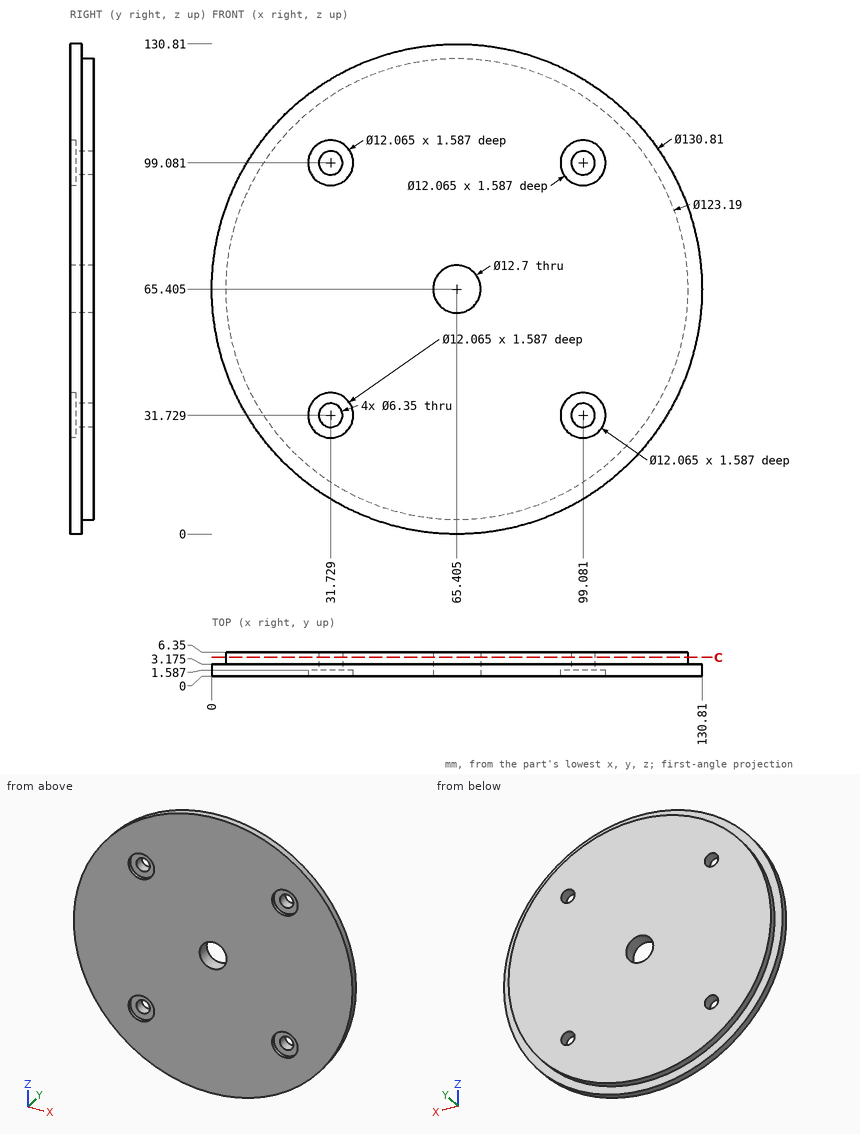
Verification items for this drawing (mm, ordinates from the low corner). Give positions to 0.01 mm unless a question says otherwise; leave off trailing zeros. Use a Markdown table: item, result.
Item 1: Section check C-C (y = 5). State how many separate pieces and enclosed holes the cut face has, and give its area (3 significant figures).
Answers follow:
| item | result |
|---|---|
| separate pieces | 1 |
| enclosed holes | 5 |
| area | 11,700 mm2 |
Item 2: Depth check by flat-ended pin: P1, Ø1.5, axis at x = 70.5, y = 4, coming from the -Z side; P2, Ø6, axis at x = 32, z = 99, coming from the -Y side. Enter the tip coordinate at first touch or a pass-through.
Answers follow:
| item | result |
|---|---|
| P1 | stops at z = 3.96 |
| P2 | stops at y = 1.59 |
Item 3: Material ranges on line 1 along Z through (x, y) = (32, 3.5) (1 decimal); line 2 along X through (y, z) = (3, 98.5); line 3 along X through (y, z) = (1.5, 64) (1 decimal), recorded low to high.
Answers follow:
| item | result |
|---|---|
| line 1 | z = 13.7 to 28.6, 34.9 to 95.9, 102.2 to 117.2 |
| line 2 | x = 8.99 to 28.61, 34.85 to 95.96, 102.2 to 121.82 |
| line 3 | x = 0 to 59.2, 71.6 to 130.8 |
